from build123d import *

# Parameters (mm, degrees)
BOX_W        = 228.5
BOX_H        = 144
BOX_DEPTH    = 26
SKETCH001_W  = 180
SKETCH001_H  = 105
POCKET_DEPTH = 26.001
FILLET_R     = 1


with BuildPart() as part:
    # Box → Box (new body)
    with BuildSketch(Plane.XY):
        with Locations((114.25, 72)):
            Rectangle(BOX_W, BOX_H)
    extrude(amount=BOX_DEPTH)

    # Sketch001 (on Face5 of Box) → Pocket (cut, through all)
    with BuildSketch(Plane(origin=(0, 0, 0), x_dir=(1, 0, 0), z_dir=(0, 0, -1))):
        with Locations((114, -66.5)):
            Rectangle(SKETCH001_W, SKETCH001_H)
    extrude(amount=-POCKET_DEPTH, mode=Mode.SUBTRACT)

    # Fillet
    fillet_edges = [part.edges().sort_by_distance(p)[0] for p in [
        (114.25, 0, 26),
    ]]
    fillet(fillet_edges, radius=FILLET_R)


solid = part.part
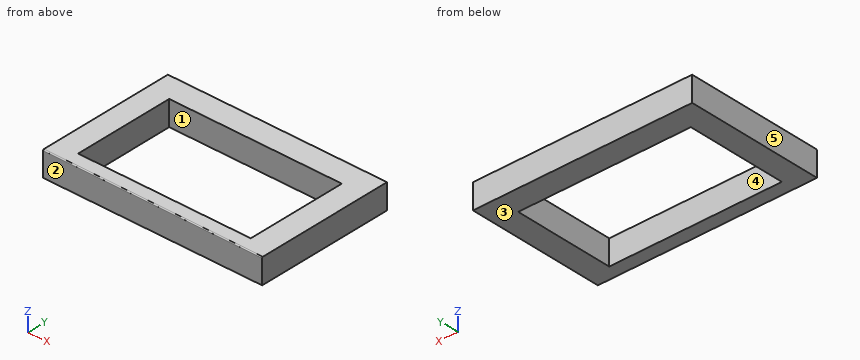
Can you work these out from the model? Positions are in its coordinate system, mm. Face numbers are marked on the shaded views. A direction names the side the tool comes from. Give positions to 0.01 mm unless a question says otherwise; leave off trailing zeros. Loops run counter-clockwise (first coordinate to the right, second up) from the corner with the lowest first, then second, coordinate; pieces in that order, holes last. Notation, with made-up numbers: (-38.75, 5.5) - (-9.75, 5.5) arc R15 cw to (-9.75, 26.5) - close; hole circle Ø11 at (18, 51.25). An arc over 180 degrees is marked (long way). Answer as a JSON object with one key per item and string values.
Q1. If I drill on L1, parallel to X at y = 54.5, z = 13.25; L2, parallel to Y at x = 88.5, z = 11.25, over which ranges is the centre line in solid material (lowest first)?
Geometry says:
{"L1": "0 to 24, 204 to 228.5", "L2": "0 to 14, 119 to 144"}
Q2. Will this pin go through, and if not, where does the flat tip stop? P1, Ø3, axis at y = 71.5, z = 8, coming from the -X side.
Geometry says:
{"P1": "x = 0"}
Q3. Imagine slicing it at A-A on y = 99. Write out the boundary of the cut face in (x, z), plus the area to 3 significant figures.
Geometry says:
{"outline": "(0, 0) - (24, 0) - (24, 26) - (0, 26) - close; (204, 0) - (228.5, 0) - (228.5, 26) - (204, 26) - close", "area": "1,260 mm²"}
Q4. Imagine slicing it at B-B on z = 14. Write out the boundary of the cut face in (x, y), plus the area to 3 significant figures.
Geometry says:
{"outline": "(0, 0) - (228.5, 0) - (228.5, 144) - (0, 144) - close; hole (24, 14) - (204, 14) - (204, 119) - (24, 119) - close", "area": "14,000 mm²"}
Q5. Imagine slicing it at C-C on x = 112. Write out the boundary of the cut face in (y, z).
Geometry says:
{"outline": "(0, 0) - (14, 0) - (14, 26) - (1, 26) arc R1 ccw to (0, 25) - close; (119, 0) - (144, 0) - (144, 26) - (119, 26) - close"}
Q6. Which directions (+Z, -Z, +X, -X, +Y, -Y) give clear straight access to the entire face, cutting with the end or side of a thin tool? Please do the marked faces 1 and 2.
Geometry says:
{"face 1": "+Z, -Z", "face 2": "+Z, -Z, +X, -X, -Y"}
Q7. If we mould it in two halves opening along X, with no side actions, what happens to the marked faces 3, 4 and 5? For each: pulls with the +X half, pulls with the -X half, needs draft (parallel to the pull), parting line crosses it, or undercut.
Geometry says:
{"face 3": "needs draft", "face 4": "undercut", "face 5": "pulls with the -X half"}
